```python
from build123d import *

# Parameters (mm, degrees)
SKETCH2_W = 2
SKETCH2_H = 1.25
SKETCH3_R = 0.25


with BuildPart() as part:
    # Sketch2 → Revolve1 (revolve)
    with BuildSketch(Plane.XY, mode=Mode.PRIVATE) as revolve1_sk:
        with Locations((1, -0.625)):
            Rectangle(SKETCH2_W, SKETCH2_H)
    revolve1 = revolve(revolve1_sk.sketch.rotate(Axis((0, 0, 0), (1, 0, 0)), 270), axis=Axis((0, 0, 0), (1, 0, 0)))

    # Sweep1: sweep along a path in Sketch1
    with BuildLine(Plane.XY) as sweep1_path:
        Line((2, 0), (2.81, 0))
        ThreePointArc((2.81, 0), (3.517106781, -0.292893219), (3.81, -1))
        Line((3.81, -1), (3.81, -4))
    # Sketch3 → Sweep1 (sweep)
    with BuildSketch(Plane(origin=(2, 0, 0), x_dir=(0, 0, -1), z_dir=(1, 0, 0))):
        Circle(SKETCH3_R)
    sweep1 = sweep(path=sweep1_path.line)

    # Mirror1: Revolve1, Sweep1 across plane
    add(revolve1.mirror(Plane.ZY))
    add(sweep1.mirror(Plane.ZY))


solid = part.part
```
Design review of the part built by this model. Coordinates are the model's own, in mm. Give positions to 0.01 mm unless a question says otherwise; leave off trailing zeros. Order: outer loops, then holes, each group sorted by start corner. A loop starts at its lowest first (then second) coordinate and runs counter-clockwise, first axis right, second up. Notation, with made-up numbers: (-35.5, 60) -> (13.5, 60) arc R23 cw to (13.5, 74) -> close; hole circle Ø9 at (52.5, -14). An arc over 180 degrees is marked (long way). Write item = value, one per line. Start each with the question number.
(1) We need section C-C on y = -3.1. Write out the cut boundary in (x, z), plus the area to 3 significant figures.
(2) For pin 1 (1.2 mm diameter, centred on y = -0.5, z = 0.5, fed in from -X); pin 2 (1.5 mm diameter, centred on x = 3, z = 0, fed in from +Y); pin 3 (1 mm diameter, centred on x = 2, z = 1, fed in from +Y), all flat-tipped, find the tip position at first contact; note any pin that passes through.
(3) We need section A-A on z = 0. Write out the cut boundary in (x, y).
(4) We need section D-D on x = -0.25. Write out the cut boundary in (y, z), plus the area to 3 significant figures.
(5) We need section B-B on x = 2.5. Write out the cut boundary in (y, z), plus the area to 3 significant figures.
(6) To check wall thickness, follow line 1 along X through (y, z) = (0.65, -0.7); line 2 along X through (y, z) = (-1.95, 0.1); line 3 along Y through (x, z) = (-1, -0.05). State the ranges of each line that lie inside material, in increasing order.
Numbers:
q1.outline = circle Ø0.5 at (-3.81, 0); circle Ø0.5 at (3.81, 0)
q1.area = 0.393 mm^2
q2.pin_1 = -4.05
q2.pin_2 = 0.25
q2.pin_3 = 1.15
q3.outline = (-4.06, -4) -> (-3.56, -4) -> (-3.56, -1) arc R0.75 cw to (-2.81, -0.25) -> (-2, -0.25) -> (-2, -1.25) -> (2, -1.25) -> (2, -0.25) -> (2.81, -0.25) arc R0.75 cw to (3.56, -1) -> (3.56, -4) -> (4.06, -4) -> (4.06, -1) arc R1.25 ccw to (2.81, 0.25) -> (2, 0.25) -> (2, 1.25) -> (-2, 1.25) -> (-2, 0.25) -> (-2.81, 0.25) arc R1.25 ccw to (-4.06, -1) -> close
q4.outline = circle Ø2.5 at (0, 0)
q4.area = 4.91 mm^2
q5.outline = circle Ø0.5 at (0, 0)
q5.area = 0.196 mm^2
q6.line_1 = -2 to 2
q6.line_2 = -4.04 to -3.58, 3.58 to 4.04
q6.line_3 = -1.25 to 1.25
